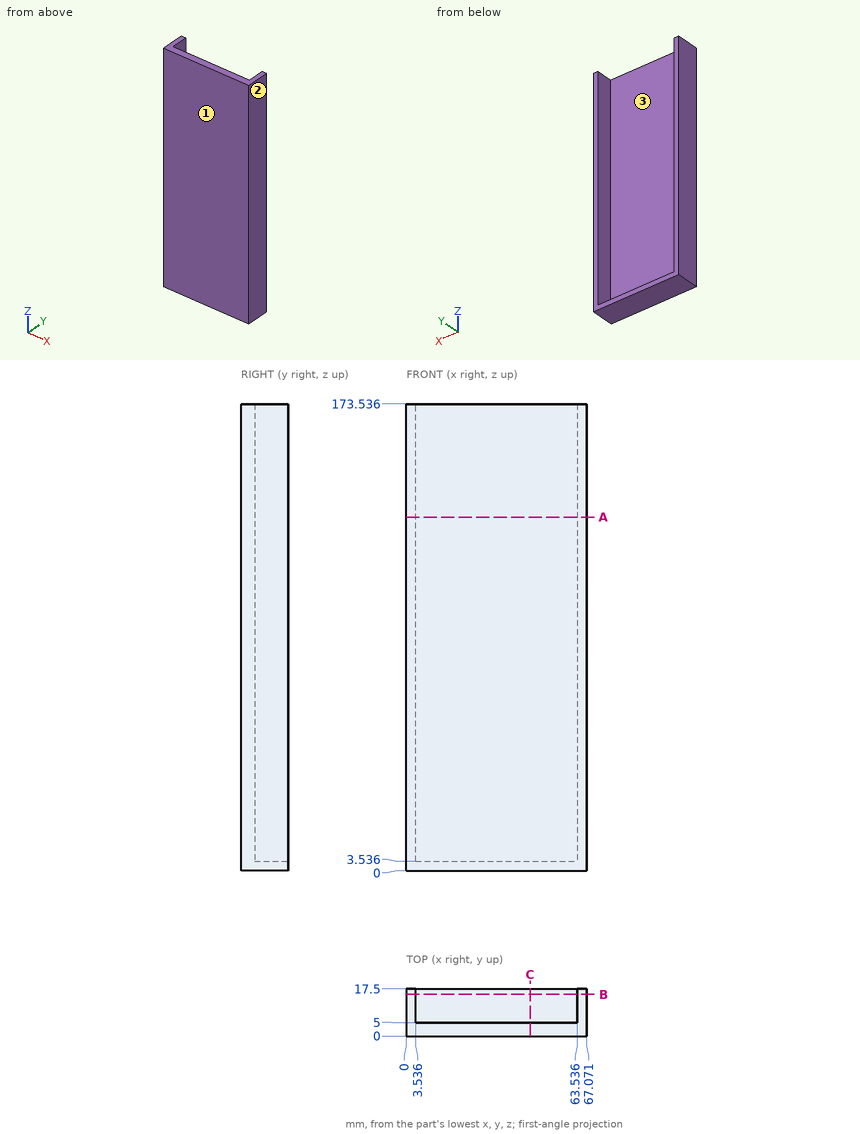
Geometry: see drawing. Coordinates: mm, zero at the bounding-box minimum. Round coordinates to 2 decimals unless told otherwise and drop trailing zeros. Write each loop counter-clockwise with the first axis right and the second up, starting at its lowest first coordinate (ties: lowest second). Pieces come first, ordered by that corner, then holes.
1) Cut plane C-C (x = 46). Return the cut outline in (y, z) (1 decimal).
2) Cut plane B-B (y = 15.5). Return the cut outline in (x, z) (1 decimal).
3) Draft query along X for the marked faces 1, 2 and 3. Return one class per face: pulls with the +X half, pulls with the -X half, needs draft (parallel to the pull), parting line crosses it, or undercut.
4) Contact query for flat-ended pins moving along their axis: P1, Ø4, axis at x = 38, y = 10.5, coming from the +Z side; P2, Ø10, axis at x = 40, z = 94.5, coming from the +Y side. Output: stop coordinate, or through.
5) Cut plane A-A (z = 131.5). Return the cut outline in (x, y) (1 decimal).
6) Ray query, L1, parallel to X at y = 15.5, z = 141.5 (1 decimal); L2, parallel to Y at x = 16, z = 31; L3, parallel to Z at x = 26.5, y = 12.5 (1 decimal). Return the intervals inside material, ascending.
Geometry says:
1. outline: (0, 0) - (17.5, 0) - (17.5, 3.5) - (5, 3.5) - (5, 173.5) - (0, 173.5) - close
2. outline: (0, 0) - (67.1, 0) - (67.1, 173.5) - (63.5, 173.5) - (63.5, 3.5) - (3.5, 3.5) - (3.5, 173.5) - (0, 173.5) - close
3. face 1: needs draft
3. face 2: pulls with the +X half
3. face 3: undercut
4. P1: stops at z = 3.54
4. P2: stops at y = 5
5. outline: (0, 0) - (67.1, 0) - (67.1, 17.5) - (63.5, 17.5) - (63.5, 5) - (3.5, 5) - (3.5, 17.5) - (0, 17.5) - close
6. L1: x = 0 to 3.5, 63.5 to 67.1
6. L2: y = 0 to 5
6. L3: z = 0 to 3.5
